from build123d import *

# Parameters (mm, degrees)
SKIZZE1_W                       = 220
SKIZZE1_H                       = 14
AUFSATZ_LINEAR_AUSTRAGEN1_DEPTH = 3
SCHNITT_LINEAR_AUSTRAGEN1_DEPTH = 111.263321191
SCHNITT_LINEAR_AUSTRAGEN2_REACH = 112.263
SKIZZE3_R                       = 1.95


with BuildPart() as part:
    # Skizze1 → Aufsatz-Linear austragen1 (new body)
    with BuildSketch(Plane(origin=(0, 0, 0), x_dir=(1, 0, 0), z_dir=(0, 1, 0))):
        Rectangle(SKIZZE1_W, SKIZZE1_H)
    extrude(amount=AUFSATZ_LINEAR_AUSTRAGEN1_DEPTH)

    # Skizze2 → Schnitt-Linear austragen1 (cut, through all)
    with BuildSketch(Plane(origin=(0, 3, 0), x_dir=(1, 0, 0), z_dir=(0, 1, 0))):
        with BuildLine():
            Line((85, 1.55), (105, 1.55))
            ThreePointArc((105, 1.55), (106.55, 0), (105, -1.55))
            Line((105, -1.55), (85, -1.55))
            ThreePointArc((85, -1.55), (83.45, 0), (85, 1.55))
        make_face()
    schnitt_linear_austragen1 = extrude(amount=-SCHNITT_LINEAR_AUSTRAGEN1_DEPTH, mode=Mode.SUBTRACT)

    # Spiegeln1: Schnitt-Linear austragen1 across plane
    add(schnitt_linear_austragen1.mirror(Plane(origin=(0, 0, 0), x_dir=(0, 0, 1), z_dir=(1, 0, 0))), mode=Mode.SUBTRACT)

    # Skizze3 → Schnitt-Linear austragen2 (cut, up to next)
    with BuildSketch(Plane(origin=(0, 3, 0), x_dir=(1, 0, 0), z_dir=(0, 1, 0)), mode=Mode.PRIVATE) as schnitt_linear_austragen2_sk1:
        with Locations(Location((27.383, 0, 0), (0, 0, 270))):
            Circle(SKIZZE3_R)
    schnitt_linear_austragen2_tool1 = extrude(schnitt_linear_austragen2_sk1.sketch, amount=-SCHNITT_LINEAR_AUSTRAGEN2_REACH, mode=Mode.PRIVATE) & part.part
    # Skizze3 → Schnitt-Linear austragen2 (cut, up to next)
    with BuildSketch(Plane(origin=(0, 3, 0), x_dir=(1, 0, 0), z_dir=(0, 1, 0)), mode=Mode.PRIVATE) as schnitt_linear_austragen2_sk2:
        with Locations(Location((62.633, 0, 0), (0, 0, 270))):
            Circle(SKIZZE3_R)
    schnitt_linear_austragen2_tool2 = extrude(schnitt_linear_austragen2_sk2.sketch, amount=-SCHNITT_LINEAR_AUSTRAGEN2_REACH, mode=Mode.PRIVATE) & part.part
    add(schnitt_linear_austragen2_tool1.solids().sort_by_distance((27.383, 3, 0))[0], mode=Mode.SUBTRACT)
    add(schnitt_linear_austragen2_tool2.solids().sort_by_distance((62.633, 3, 0))[0], mode=Mode.SUBTRACT)


solid = part.part
Can you work these out from the model? Positions are in its coordinate system, mm. Round coordinates to 2 decimals unless told otherwise and drop trailing zeros. Loops run counter-clockwise (first coordinate to the right, second up) from the corner with the lowest first, then second, coordinate; pieces in that order, holes last. Notation, with made-up numbers: (20, -12) - (47, -12) arc R4 cw to (47, -7) - close; hole circle Ø9 at (-30, 88). An arc over 180 degrees is marked (long way). Write item = value, one per line. Start each with the question number.
(1) If we mould it in two halves opening along X, with no side actions, what happens to faces 1 (the face through (64.566, 1.521, -0.254)), 2 (the face through (-2, 0, 0))? For each: released by +X, released by -X, zero draft, split by the parting line, or undercut.
(2) If I drill on probe 1 along X at (y, z) = (1.7, 0); probe 2 along X at (y, z) = (0.9, -0.5); probe 3 along Z at (x, y) = (90, 2.2), over which ranges is the centre line in solid material (lowest first)? Write a range as [from, to].
(3) If we section it at A-A (y = 2.05): Please give me the cut outline in (x, z).
Ans:
q1.face_1 = undercut
q1.face_2 = zero draft
q2.probe_1 = [-110, -106.55], [-83.45, 25.43], [29.33, 60.68], [64.58, 83.45], [106.55, 110]
q2.probe_2 = [-110, -106.47], [-83.53, 25.5], [29.27, 60.75], [64.52, 83.53], [106.47, 110]
q2.probe_3 = [-7, -1.55], [1.55, 7]
q3.outline = (-110, -7) - (110, -7) - (110, 7) - (-110, 7) - close; hole (-105, -1.55) - (-85, -1.55) arc R1.55 ccw to (-85, 1.55) - (-105, 1.55) arc R1.55 ccw to start; hole circle Ø3.9 at (27.38, 0); hole circle Ø3.9 at (62.63, 0); hole (85, -1.55) - (105, -1.55) arc R1.55 ccw to (105, 1.55) - (85, 1.55) arc R1.55 ccw to start
